Geometry check sheet. Reference: the model listing, model coordinates, mm. Face numbers are marked on the shaded views. A direction names the side the tool comes from. Round coordinates to 2 decimals unless told otherwise and drop trailing zeros. Order: outer loops, then holes, each group sorted by start corner. A loop starts at its lowest first (then second) coordinate and runs counter-clockwise, first axis right, second up. Notation, with made-up numbers: (20, -4.75) - (27, -4.75) arc R22 cw to (27, 3.25) - close; hole circle Ø7 at (62, 41). An arc over 180 degrees is marked (long way). Answer as CSV lines item,"result". Start each with the question number.
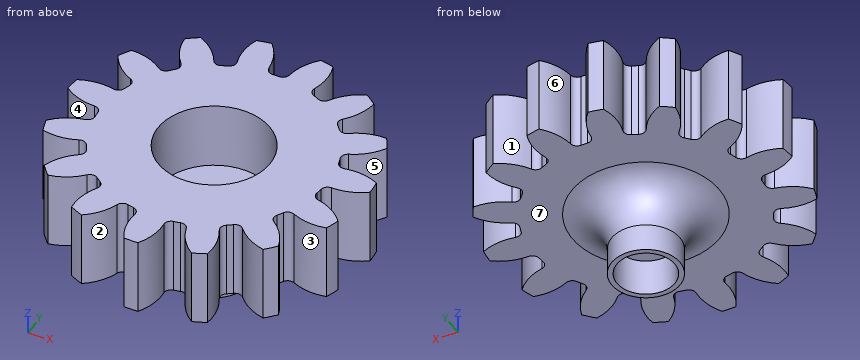
```python
from build123d import *

# Parameters (mm, degrees)
SKETCH3_R          = 21.59
GEARBODY_DEPTH     = 11
TOOTHCUT_DEPTH     = 12
CIRPATTERN1_COUNT  = 15
BOREDIA_R          = 7.874
BORE_DEPTH         = 12700
SKETCH6_R          = 4.1
CUT_EXTRUDE1_DEPTH = 5.3


with BuildPart() as part:
    # Sketch3 → gearBody (new body)
    with BuildSketch(Plane.XY):
        Circle(SKETCH3_R)
    extrude(amount=GEARBODY_DEPTH)

    # Sketch2 → toothCut (cut, through all)
    with BuildSketch(Plane.XY):
        with BuildLine():
            ThreePointArc((15.783846764, -2.304552616), (15.843293638, -1.852249483), (15.889781974, -1.39843136))
            ThreePointArc((15.889781974, -1.39843136), (16.213055843, -0.751556907), (16.890861518, -0.499501321))
            ThreePointArc((16.890861518, -0.499501321), (20.504912911, 0.340315353), (23.283949955, 2.798691365))
            ThreePointArc((23.283949955, 2.798691365), (23.292901215, -2.723187818), (22.010467945, -8.09409042))
            ThreePointArc((22.010467945, -8.09409042), (19.873444675, -5.060974685), (16.550574786, -3.410158156))
            ThreePointArc((16.550574786, -3.410158156), (15.949189176, -3.008551507), (15.783846764, -2.304552616))
        make_face()
    toothcut = extrude(amount=TOOTHCUT_DEPTH, mode=Mode.SUBTRACT)

    # CirPattern1: toothCut ×15 about axis
    cirpattern1_axis = Axis((0, 0, 0), (0, 0, 1))
    for i in range(1, CIRPATTERN1_COUNT):
        add(toothcut.rotate(cirpattern1_axis, i * 360 / CIRPATTERN1_COUNT), mode=Mode.SUBTRACT)

    # boreDia → bore (cut, symmetric)
    with BuildSketch(Plane.XY):
        Circle(BOREDIA_R)
    extrude(amount=BORE_DEPTH, both=True, mode=Mode.SUBTRACT)

    # Sketch4 → Revolve1 (revolve)
    with BuildSketch(Plane(origin=(0, 0, 0), x_dir=(0, 0, -1), z_dir=(1, 0, 0))):
        with BuildLine():
            Line((0, 0), (9.525, 0))
            Line((9.525, 0), (9.525, 4.826))
            Line((9.525, 4.826), (5.588, 4.826))
            ThreePointArc((5.588, 4.826), (1.636687307, 6.462687307), (0, 10.414))
            Line((0, 10.414), (0, 7.874))
            Line((0, 7.874), (-1.524, 7.874))
            Line((-1.524, 7.874), (-1.524, 0))
            Line((-1.524, 0), (0, 0))
        make_face()
    revolve(axis=Axis((0, 0, 0), (0, 0, -1)))

    # Sketch6 → Cut-Extrude1 (cut)
    with BuildSketch(Plane(origin=(0, 0, -9.525), x_dir=(-1, 0, 0), z_dir=(0, 0, -1))):
        Circle(SKETCH6_R)
    extrude(amount=-CUT_EXTRUDE1_DEPTH, mode=Mode.SUBTRACT)


solid = part.part
```
1. Section check A-A on z = -6.75. Record the boundary of the cut face in (x, y), plus the area to 3 significant figures.
2. Draft check along X on the marked faces 5, 6 and 7. Enter one of: released by +X, released by -X, zero draft, split by the parting line, or undercut.
3. Go/stop test with flat-tipped pins: pin 1 Ø1.5 at (y, z) = (16, 4.5) entering from +X; pin 2 Ø5 at (x, z) = (17, 1) entering from -Y; pin 3 Ø6 at (y, z) = (-13.5, 7.5) entering from -X. Record where each tip stops, or that it passes through.
4. Section check B-B on z = -3. Record the boundary of the cut face in (x, y).
5. Thickness scan on probe 1 along Y at (x, z) = (15.5, 6.75); probe 2 along X at (y, z) = (-14, 6); probe 3 along Y at (x, z) = (-18.5, 9.75). Record the ranges inside material, lowest first.
6. Access from +Z, -Z, +X, -X, +Y, -Y to the whole of each face (thin tool, end or side, straight path). Record for the marked faces 1, 2, 3 and 4.
Numbers:
1,outline,"circle Ø9.65 at (0, 0); hole circle Ø8.2 at (0, 0)"
1,area,"20.4 mm2"
2,face 5,"released by +X"
2,face 6,"undercut"
2,face 7,"zero draft"
3,pin 1,"stops at x = 13.68"
3,pin 2,"stops at y = -15.35"
3,pin 3,"stops at x = -16.86"
4,outline,"circle Ø10.92 at (0, 0)"
5,probe 1,"y = -15.03 to -11.67, -7.45 to 4.01, 6.34 to 11.01"
5,probe 2,"x = -16.44 to -12.89, -8.74 to 8.41, 12.13 to 16.44"
5,probe 3,"y = -7.61 to -3.65, 0.07 to 4.19, 9.23 to 11.13"
6,face 1,"+Z, -Z, +Y"
6,face 2,"+Z, -Z, -Y"
6,face 3,"+Z, -Z"
6,face 4,"+Z, -Z, -X"
